The figure shows three views and two pictorial views of one solid part (mm, origin at its lowest corner). Answer the questions. Coordinates: 2 decimals unless noted, no trailing zeros. Loops run counter-clockwise (first coordinate to the right, second up) from the corner with the lowest first, then second, coordinate; pieces in that order, holes last. Notation, with made-up numbers: M 51,53.5 L 89,53.5 A16 cw 89,58.5 Z; hole C 88,42.5 d10. An arc over 180 degrees is marked long. Write each question's results on one line, items separated by ' | '.
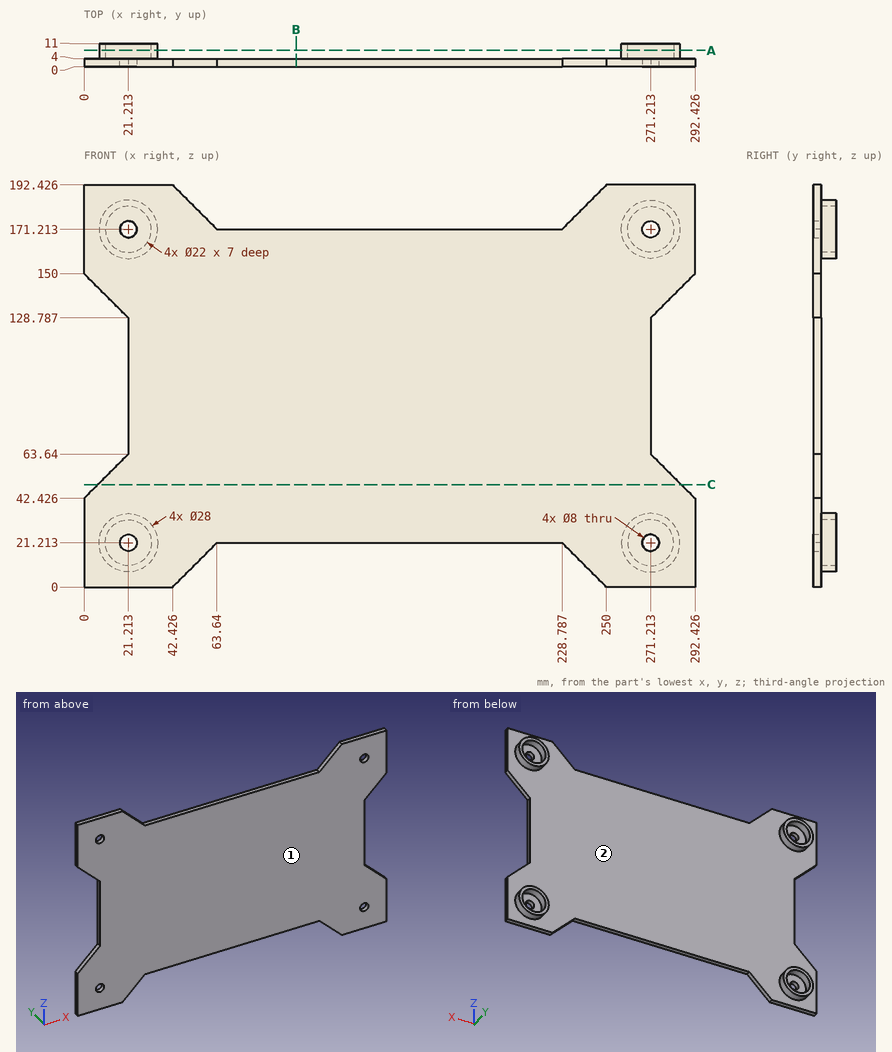
1) Straight lines are drawn through the part: probe 1 along X at (y, z) = (10.25, 162) (1 decimal); probe 2 along Y at (x, z) = (158, 56); probe 3 along X at (y, z) = (3, 123). For each, find the intervals that lie inside material, in ascending order. Write a range as [from, to].
Check result:
probe 1: [10.7, 15.2], [27.2, 31.8], [260.7, 265.2], [277.2, 281.8] | probe 2: [0, 4] | probe 3: [21.21, 271.21]
2) Find section A-A, the plane y = 8. Give the vertices of the cut face in (x, z).
Check result:
outline: C 21.21,21.21 d28; C 21.21,171.21 d28; C 271.21,21.21 d28; C 271.21,171.21 d28; hole C 21.21,21.21 d22; hole C 21.21,171.21 d22; hole C 271.21,21.21 d22; hole C 271.21,171.21 d22
3) Find section C-C, the plane z = 49. Give the vertices of the cut face in (x, y), and give its area (3 significant figures).
Check result:
outline: M 6.57,0 L 285.85,0 L 285.85,4 L 6.57,4 Z | area: 1,120 mm^2
4) Find section B-B, the plane x = 101.5. Give the vertices of the cut face in (y, z), and give its area (3 significant figures).
Check result:
outline: M 0,21.21 L 4,21.21 L 4,171.21 L 0,171.21 Z | area: 600 mm^2
5) For a pull along X with two mould halves and no side action, classify the marked faces 1 and 2 as released by +X, released by -X, zero draft, split by the parting line, or undercut.
Check result:
face 1: zero draft | face 2: undercut
6) Given pin 1 Ø6.5 at (x, z) = (23.5, 168) entering from +Y; pin 2 Ø4.5 at (y, z) = (1.5, 94) entering from +X; pin 3 Ø1.2 at (x, y) = (168, 3) entering from +Z, each flat-ended and moving along its own axis, determine where each tip first touches the part or whether it passes through.
Check result:
pin 1: y = 4 | pin 2: x = 271.21 | pin 3: z = 171.21
